Can you work these out from the model? Positions are in its coordinate system, mm. A direction names the side the tool comes from. Give positions to 0.01 mm unless a question says otherwise; leave off trailing zeros. Loops run counter-clockwise (first coordinate to the right, second up) from the corner with the lowest first, then second, coordinate; pieces in that order, holes last. Notation, with made-up numbers: M -19,85.25 L 7,85.25 A26 ccw 7,124.25 Z; hole C 83.5,-17 d9. An arc over 180 degrees is marked long. Use CSV: the item, a comma, the result in double quotes.
from build123d import *

# Parameters (mm, degrees)
BOSS_EXTRUDE1_DEPTH     = 6
SKETCH4_R               = 1.75
SERVO_HORN_HOLES_DEPTH  = 29.222331583
SKETCH5_R               = 8
BEARING_PRESS_FIT_DEPTH = 4.5
SKETCH7_R               = 12.5
CUT_EXTRUDE1_DEPTH      = 3
SKETCH8_R               = 7
CUT_EXTRUDE2_DEPTH      = 28.941904015


with BuildPart() as part:
    # Sketch2 → Boss-Extrude1 (new body)
    with BuildSketch(Plane(origin=(0, 0, 0), x_dir=(1, 0, 0), z_dir=(0, 1, 0))):
        with BuildLine():
            Line((15, 10.5), (-15, 10.5))
            ThreePointArc((-15, 10.5), (-25.5, 0), (-15, -10.5))
            Line((-15, -10.5), (15, -10.5))
            ThreePointArc((15, -10.5), (25.5, 0), (15, 10.5))
        make_face()
    extrude(amount=BOSS_EXTRUDE1_DEPTH)

    # Sketch4 → Servo horn holes (cut, through all)
    with BuildSketch(Plane(origin=(0, 6, 0), x_dir=(1, 0, 0), z_dir=(0, 1, 0))):
        with Locations(Location((-15, 0, 0), (0, 0, 270))):
            Circle(SKETCH4_R)
        with Locations(Location((-8, 0, 0), (0, 0, 270))):
            Circle(SKETCH4_R)
        with Locations(Location((-15, -7, 0), (0, 0, 270))):
            Circle(SKETCH4_R)
        with Locations(Location((-22, 0, 0), (0, 0, 270))):
            Circle(SKETCH4_R)
        with Locations(Location((-15, 7, 0), (0, 0, 270))):
            Circle(SKETCH4_R)
    extrude(amount=-SERVO_HORN_HOLES_DEPTH, mode=Mode.SUBTRACT)

    # Sketch5 → Bearing press fit (cut)
    with BuildSketch(Plane(origin=(0, 0, 0), x_dir=(-1, 0, 0), z_dir=(0, -1, 0))):
        with Locations(Location((-15, 0, 0), (0, 0, 90))):
            Circle(SKETCH5_R)
    extrude(amount=-BEARING_PRESS_FIT_DEPTH, mode=Mode.SUBTRACT)

    # Sketch7 → Cut-Extrude1 (cut)
    with BuildSketch(Plane(origin=(0, 6, 0), x_dir=(1, 0, 0), z_dir=(0, 1, 0))):
        with Locations((-15, 0)):
            Circle(SKETCH7_R)
    extrude(amount=-CUT_EXTRUDE1_DEPTH, mode=Mode.SUBTRACT)

    # Sketch8 → Cut-Extrude2 (cut, through all)
    with BuildSketch(Plane.XZ.offset(-4.5)):
        with Locations(Location((15, 0, 0), (0, 0, 270))):
            Circle(SKETCH8_R)
    extrude(amount=-CUT_EXTRUDE2_DEPTH, mode=Mode.SUBTRACT)


solid = part.part
Q1. If we mould it in two halves opening along Z, with no side actions, what happens to faces 4 (the flat face through (0, 3, 10.5)), 5 (the flat face through (-14, 3, 2)), 6 (the flat face through (8, 6, -2)), 7 (the cylindrical face through (-13.265, 1.521, 6.772))? For each: released by +Z, released by -Z, zero draft, split by the parting line, or undercut.
Model answer:
face 4,"released by +Z"
face 5,"undercut"
face 6,"zero draft"
face 7,"undercut"
Q2. For faces 1 (the flat face through (9, 4.5, -4)), 2 (the flat face through (0, 3, -10.5)), 3 (the cylindrical face through (-2.5, 4.5, 0.2)), which set-ups out of +Z, -Z, +X, -X, +Y, -Y let a thin tool reach every point of the face, with its end or its side?
Model answer:
face 1,"-Y"
face 2,"-Z, +X, -X, +Y, -Y"
face 3,"-X, +Y"
Q3. I want a section at D-D, the plane x = 19.5. Please give me the cut outline in (y, z).
Model answer:
outline,"M 0,-9.49 L 6,-9.49 L 6,-5.36 L 4.5,-5.36 L 4.5,-6.61 L 0,-6.61 Z; M 0,6.61 L 4.5,6.61 L 4.5,5.36 L 6,5.36 L 6,9.49 L 0,9.49 Z"
Q4. I want a section at A-A, the plane z = 0. Please give me the cut outline in (x, y), then the cut area to 4 significant figures.
Model answer:
outline,"M -25.5,0 L -23.75,0 L -23.75,3 L -25.5,3 Z; M -20.25,0 L -16.75,0 L -16.75,3 L -20.25,3 Z; M -13.25,0 L -9.75,0 L -9.75,3 L -13.25,3 Z; M -6.25,0 L 7,0 L 7,4.5 L 8,4.5 L 8,6 L -2.5,6 L -2.5,3 L -6.25,3 Z; M 22,4.5 L 23,4.5 L 23,0 L 25.5,0 L 25.5,6 L 22,6 Z"
area,"112.5 mm2"
Q5. I want a section at B-B, the plane y = 0.85. Please give me the cut outline in (x, z).
Model answer:
outline,"M -15,-10.5 L 15,-10.5 A10.5 ccw 15,10.5 L -15,10.5 A10.5 ccw Z; hole C -22,0 d3.5; hole C -15,-7 d3.5; hole C -15,0 d3.5; hole C -15,7 d3.5; hole C -8,0 d3.5; hole C 15,0 d16"
Q6. I'm going to push flat-ended pins straight in: P1, Ø2, axis at x = -12.5, z = 1.5, coming from the +Y side; P2, Ø2, axis at y = 3, z = 2, coming from the -X side. Where does each tip first touch, or does it pass through?
Model answer:
P1,"y = 3"
P2,"x = -25.45"
Q7. I want a section at C-C, the plane y = 3.9. Please give me the cut outline in (x, z), then the cut area to 3 significant figures.
Model answer:
outline,"M -8.22,-10.5 L 15,-10.5 A10.5 ccw 15,10.5 L -8.22,10.5 A12.5 cw Z; hole C 15,0 d16"
area,"375 mm2"
Q8. Please list where these lines run through material, in increasing order: L1, parallel to X at y = 2.4, z = 0; L2, parallel to X at y = 4.95, z = 0.25; L3, parallel to X at y = 1.95, z = -7. Write a range as from..to.
Model answer:
L1,"-25.5..-23.75, -20.25..-16.75, -13.25..-9.75, -6.25..7, 23..25.5"
L2,"-2.5..8, 22..25.5"
L3,"-22.83..-16.75, -13.25..11.13, 18.87..22.83"
